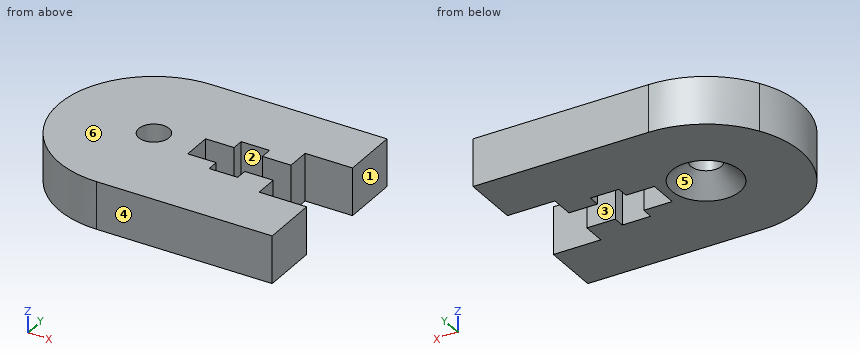
from build123d import *

# Parameters (mm, degrees)
BOSS_EXTRU_1_DEPTH                  = 5
ESQUISSE2_W                         = 5
ESQUISSE2_H                         = 8
ENL_V_MAT_EXTRU_1_DEPTH             = 6
ENL_V_MAT_EXTRU_2_DEPTH             = 2.5
DIAM_TRE_DU_PER_AGE_2_5_2_5_2_D     = 2.5
DIAM_TRE_DU_PER_AGE_2_5_2_5_2_DEPTH = 2.5
ESQUISSE9_W                         = 8.5
ESQUISSE9_H                         = 10
BOSS_EXTRU_2_DEPTH                  = 5
ESQUISSE10_R                        = 1.6
ESQUISSE10_W                        = 9
ESQUISSE10_H                        = 3.1
ESQUISSE10_W_2                      = 3
ESQUISSE10_H_2                      = 5.55
ENL_V_MAT_EXTRU_3_DEPTH             = 6
CHANFREIN1_SIZE                     = 2


with BuildPart() as part:
    # Esquisse1 → Boss.-Extru.1 (new body)
    with BuildSketch(Plane(origin=(0, 0, 0), x_dir=(-1, 0, 0), z_dir=(0, 0, -1))):
        with BuildLine():
            Line((-17, 10), (-17, -10))
            Line((-17, -10), (1.5, -10))
            ThreePointArc((1.5, -10), (11.5, 0), (1.5, 10))
            Line((1.5, 10), (-17, 10))
        make_face()
    extrude(amount=-BOSS_EXTRU_1_DEPTH)

    # Esquisse2 → Enlèv. mat.-Extru.1 (cut, through all)
    with BuildSketch(Plane.XY.offset(5)):
        with Locations((14.5, 0)):
            Rectangle(ESQUISSE2_W, ESQUISSE2_H)
    extrude(amount=-ENL_V_MAT_EXTRU_1_DEPTH, mode=Mode.SUBTRACT)

    # Esquisse3 → Enlèv. mat.-Extru.2 (cut)
    with BuildSketch(Plane.XY.offset(5)):
        with BuildLine():
            Line((-10.160254038, -5), (7, -5))
            Line((7, -5), (7, 5))
            Line((7, 5), (-10.160254038, 5))
            ThreePointArc((-10.160254038, 5), (-11.5, 0), (-10.160254038, -5))
        make_face()
    extrude(amount=-ENL_V_MAT_EXTRU_2_DEPTH, mode=Mode.SUBTRACT)

    # Diamètre du perçage Ø2.5 (2.5)2
    with Locations(Plane.XY.offset(2.5)):
        with Locations((-1.5, 0)):
            Hole(DIAM_TRE_DU_PER_AGE_2_5_2_5_2_D / 2, depth=DIAM_TRE_DU_PER_AGE_2_5_2_5_2_DEPTH)

    # Esquisse9 → Boss.-Extru.2 (add)
    with BuildSketch(Plane.XY.offset(5)):
        with BuildLine():
            Line((-10.160254038, -5), (-1.5, -5))
            Line((-1.5, -5), (-1.5, 5))
            Line((-1.5, 5), (-10.160254038, 5))
            ThreePointArc((-10.160254038, 5), (-11.5, 0), (-10.160254038, -5))
        make_face()
        with Locations((2.75, 0)):
            Rectangle(ESQUISSE9_W, ESQUISSE9_H)
    extrude(amount=-BOSS_EXTRU_2_DEPTH)

    # Esquisse10 → Enlèv. mat.-Extru.3 (cut, through all)
    with BuildSketch(Plane.XY.offset(5)):
        with Locations((-1.5, 0)):
            Circle(ESQUISSE10_R)
        with Locations((7.5, 0)):
            Rectangle(ESQUISSE10_W, ESQUISSE10_H)
        with Locations((7.5, 0.005)):
            Rectangle(ESQUISSE10_W_2, ESQUISSE10_H_2)
    extrude(amount=-ENL_V_MAT_EXTRU_3_DEPTH, mode=Mode.SUBTRACT)

    # Chanfrein1
    chanfrein1_edges = [part.edges().sort_by_distance(p)[0] for p in [
        (-3.1, 0, 0),
    ]]
    chamfer(chanfrein1_edges, length=CHANFREIN1_SIZE)


solid = part.part
Input: part model. Units: mm. Frame: model coordinates. Face numbers are marked on the shaded views. A direction names the side the tool comes from. Give positions to 0.01 mm unless a question says otherwise; leave off trailing zeros. Write each loop counter-clockwise with the first axis right and the second up, starting at its lowest first coordinate (ties: lowest second). Pieces come first, ordered by that corner, then holes. Notation, with made-up numbers: (-11.5, 35) -> (17.5, 35) arc R16 cw to (17.5, 39) -> close; hole circle Ø4 at (6, 75.25). An arc over 180 degrees is marked (long way). Use one line per item in the form item = value. Start each with the question number.
1) Set-up query: the marked faces 1, 2 and 3. Return all of +Z, -Z, +X, -X, +Y, -Y with unobstructed straight access to the full face (end or side cutting, diameter ignored); none if empty.
2) Section query C-C on y = 0. Return the cut outline in (x, z), then the cut area to 3 significant figures.
3) Pin query (flat end, axial travel): pin 1 (0.6 mm diameter, centred on y = -2, z = 2.5, fed in from +X); pin 2 (1 mm diameter, centred on y = -2, z = 3, fed in from -X); pin 3 (5 mm diameter, centred on x = -1.5, y = 0, fed in from -Z). Return the tip coordinate at first contact, or that it passes through.
4) Section query B-B on x = 10.5. Return the cut outline in (y, z), then the cut area to 3 significant figures.
5) Section query D-D on y = -6. Return the cut outline in (x, z), then the cut area to 4 significant figures.
6) Section query A-A on z = 1. Return the cut outline in (x, y).
7) Draft query along Y for the marked faces 4, 5 and 6. Return one class per face: pulls with the +Y half, pulls with the -Y half, needs draft (parallel to the pull), parting line crosses it, or undercut.
8) Ray query, probe 1 along Y at (x, z) = (3.75, 1.8); probe 2 along Y at (x, z) = (7, 4.7); probe 3 along X at (y, z) = (0.5, 0.5). Return the intervals inside material, ascending. Write a range as from..to.
Outcome:
q1.face_1 = +Z, -Z, +X, +Y, -Y
q1.face_2 = +Z, -Z
q1.face_3 = +Z, -Z, +X
q2.outline = (-11.5, 0) -> (-5.1, 0) -> (-3.1, 2) -> (-3.1, 5) -> (-11.5, 5) -> close; (0.1, 2) -> (2.1, 0) -> (3, 0) -> (3, 5) -> (0.1, 5) -> close
q2.area = 52.5 mm^2
q3.pin_1 = 12
q3.pin_2 = -11.39
q3.pin_3 = 1.1
q4.outline = (-10, 0) -> (-1.55, 0) -> (-1.55, 5) -> (-10, 5) -> close; (1.55, 0) -> (10, 0) -> (10, 5) -> (1.55, 5) -> close
q4.area = 84.5 mm^2
q5.outline = (-9.5, 0) -> (17, 0) -> (17, 5) -> (-9.5, 5) -> close
q5.area = 132.5 mm^2
q6.outline = (-1.5, -10) -> (17, -10) -> (17, -4) -> (12, -4) -> (12, -1.55) -> (9, -1.55) -> (9, -2.77) -> (6, -2.77) -> (6, -1.55) -> (3, -1.55) -> (3, 1.55) -> (6, 1.55) -> (6, 2.78) -> (9, 2.78) -> (9, 1.55) -> (12, 1.55) -> (12, 4) -> (17, 4) -> (17, 10) -> (-1.5, 10) arc R10 ccw to start; hole circle Ø5.2 at (-1.5, 0)
q7.face_4 = pulls with the -Y half
q7.face_5 = undercut
q7.face_6 = needs draft
q8.probe_1 = -10..-1.55, 1.55..10
q8.probe_2 = -10..-2.77, 2.78..10
q8.probe_3 = -11.49..-4.56, 1.56..3
